For this review, take the finished solid that the model builds, in its own axes (mm). Face numbers are marked on the shaded views. A direction names the side the tool comes from. Coordinates: 2 decimals unless noted, no trailing zeros. Order: outer loops, then holes, each group sorted by start corner. A loop starts at its lowest first (then second) coordinate and runs counter-clockwise, first axis right, second up.
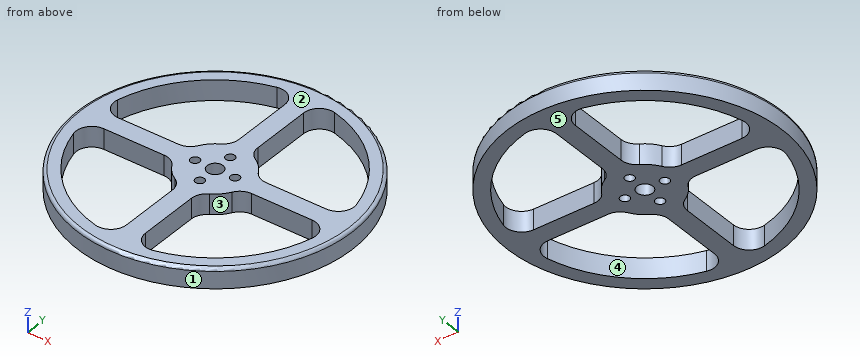
from build123d import *

# Parameters (mm, degrees)
F0_R     = 43.5
F0_R_2   = 1.45
F0_R_3   = 2.5
F1_DEPTH = 6.4
F2_R     = 5
F3_R     = 1


with BuildPart() as f1:
    # F0 (on Top) → F1 (new body)
    with BuildSketch(Plane.XY):
        Circle(F0_R)
        with BuildLine():
            ThreePointArc((-10.608988, -3), (-7.795852, -7.795852), (-3, -10.608988))
            Line((-3, -10.608988), (-3, -38.884444))
            ThreePointArc((-3, -38.884444), (-27.577164, -27.577164), (-38.884444, -3))
            Line((-38.884444, -3), (-10.608988, -3))
        make_face(mode=Mode.SUBTRACT)
        with BuildLine():
            ThreePointArc((3, -10.608988), (7.795852, -7.795852), (10.608988, -3))
            Line((10.608988, -3), (38.884444, -3))
            ThreePointArc((38.884444, -3), (27.577164, -27.577164), (3, -38.884444))
            Line((3, -38.884444), (3, -10.608988))
        make_face(mode=Mode.SUBTRACT)
        with Locations((0, -6.35)):
            Circle(F0_R_2, mode=Mode.SUBTRACT)
        with Locations((-6.35, 0)):
            Circle(F0_R_2, mode=Mode.SUBTRACT)
        with BuildLine():
            ThreePointArc((-3, 10.608988), (-7.795852, 7.795852), (-10.608988, 3))
            Line((-10.608988, 3), (-38.884444, 3))
            ThreePointArc((-38.884444, 3), (-27.577164, 27.577164), (-3, 38.884444))
            Line((-3, 38.884444), (-3, 10.608988))
        make_face(mode=Mode.SUBTRACT)
        Circle(F0_R_3, mode=Mode.SUBTRACT)
        with Locations((6.35, 0)):
            Circle(F0_R_2, mode=Mode.SUBTRACT)
        with Locations((0, 6.35)):
            Circle(F0_R_2, mode=Mode.SUBTRACT)
        with BuildLine():
            ThreePointArc((10.608988, 3), (7.795852, 7.795852), (3, 10.608988))
            Line((3, 10.608988), (3, 38.884444))
            ThreePointArc((3, 38.884444), (27.577164, 27.577164), (38.884444, 3))
            Line((38.884444, 3), (10.608988, 3))
        make_face(mode=Mode.SUBTRACT)
    extrude(amount=F1_DEPTH)

    # F2
    f2_edges = [f1.edges().sort_by_distance(p)[0] for p in [
        (-10.608988, -3, 3.2),
        (-3, -10.608988, 3.2),
        (-3, 10.608988, 3.2),
        (-10.608988, 3, 3.2),
        (3, -10.608988, 3.2),
        (10.608988, -3, 3.2),
        (10.608988, 3, 3.2),
        (3, 10.608988, 3.2),
        (-38.884444, -3, 3.2),
        (-3, -38.884444, 3.2),
        (3, -38.884444, 3.2),
        (38.884444, -3, 3.2),
        (38.884444, 3, 3.2),
        (3, 38.884444, 3.2),
        (-3, 38.884444, 3.2),
        (-38.884444, 3, 3.2),
    ]]
    fillet(f2_edges, radius=F2_R)

    # F3
    f3_edges = [f1.edges().sort_by_distance(p)[0] for p in [
        (-43.5, 0, 6.4),
    ]]
    fillet(f3_edges, radius=F3_R)


solid = f1.part
1. To check wall thickness, follow L1, parallel to Y at x = 0, z = 1.75; L2, parallel to Y at x = -19, z = 4; L3, parallel to Y at x = -36, z = 2.5. State the ranges of each line that lie inside material, in increasing order.
Answer below:
L1: y = -43.5 to -7.8, -4.9 to -2.5, 2.5 to 4.9, 7.8 to 43.5
L2: y = -39.13 to -34.06, -3 to 3, 34.06 to 39.13
L3: y = -24.42 to -15, -3.97 to 3.97, 15 to 24.42
2. Clearance check with flat-ended pins moving along their axes: pin 1 Ø1.7 at (x, y) = (6.35, 0) entering from +Z; pin 2 Ø4 at (x, y) = (0, -6.35) entering from -Z; pin 3 Ø3 at (y, z) = (-20.5, 3) entering from -X; pin 4 Ø3 at (x, z) = (24.5, 3.5) entering from +Y. State where each tip first meets the part, or that it passes through.
Answer below:
pin 1: passes through
pin 2: stops at z = 0
pin 3: stops at x = -39.13
pin 4: stops at y = 36.92
3. The part is to be moulded in two halves that separate along X. For the marked faces 1, 2 and 3, say which applies: +X half, -X half, draft (parallel to the pull), parting line (faces both ways), or undercut.
Answer below:
face 1: parting line
face 2: draft
face 3: undercut
4. Take a section at A-A, the plane x = 0. Give the boundary of the cut face in (y, z).
Answer below:
outline: (-43.5, 0) - (-7.8, 0) - (-7.8, 6.4) - (-42.5, 6.4) arc R1 ccw to (-43.5, 5.4) - close; (-4.9, 0) - (-2.5, 0) - (-2.5, 6.4) - (-4.9, 6.4) - close; (2.5, 0) - (4.9, 0) - (4.9, 6.4) - (2.5, 6.4) - close; (7.8, 0) - (43.5, 0) - (43.5, 5.4) arc R1 ccw to (42.5, 6.4) - (7.8, 6.4) - close
5. Take a section at C-C, the plane z = 1.75. Give the number of separate pieces and of enclosed holes in the cut face, plus the area to 3 significant figures.
Answer below:
separate pieces: 1
enclosed holes: 9
area: 2,250 mm2
6. Machinability: for the marked faces 4 and 5, which of the approach directions +Z, -Z, +X, -X, +Y, -Y give a long, thin tool a straight path to every point of the face, cutting with its end or side? Answer none if there is none.
Answer below:
face 4: +Z, -Z
face 5: -Z, +X, -X, +Y, -Y
